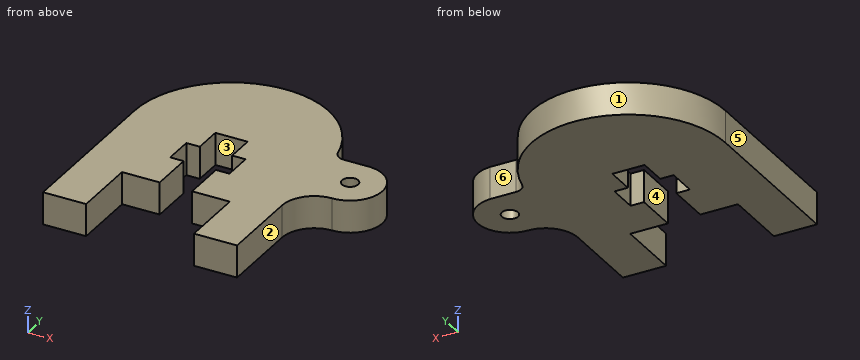
from build123d import *

# Parameters (mm, degrees)
SKETCH_1_R      = 0.75
EXTRUDE_1_DEPTH = 3


with BuildPart() as part:
    # 草图1 → 凸台-拉伸1 (new body)
    with BuildSketch(Plane.XY):
        with BuildLine():
            Line((0, 0), (4, 0))
            Line((4, 0), (4, 6))
            Line((4, 6), (7.5, 6))
            Line((7.5, 6), (7.5, 10))
            Line((7.5, 10), (6.25, 10))
            Line((6.25, 10), (6.25, 12.7))
            Line((6.25, 12.7), (7.5, 12.7))
            Line((7.5, 12.7), (7.5, 15.3))
            Line((7.5, 15.3), (10.5, 15.3))
            Line((10.5, 15.3), (10.5, 12.7))
            Line((10.5, 12.7), (11.75, 12.7))
            Line((11.75, 12.7), (11.75, 10))
            Line((11.75, 10), (10.5, 10))
            Line((10.5, 10), (10.5, 6))
            Line((10.5, 6), (14, 6))
            Line((14, 6), (14, 0))
            Line((14, 0), (18, 0))
            Line((18, 0), (18, 7.5))
            ThreePointArc((18, 7.5), (18.878679656, 9.621320344), (21, 10.5))
            ThreePointArc((21, 10.5), (23.998598833, 13.408321005), (21.183272352, 16.494396641))
            Line((21.183272352, 16.494396641), (18.756260727, 16.494396641))
            ThreePointArc((18.756260727, 16.494396641), (18.131536654, 16.713551053), (17.780634655, 17.274956977))
            ThreePointArc((17.780634655, 17.274956977), (8.006448766, 24.24499055), (0, 15.3))
            Line((0, 15.3), (0, 0))
        make_face()
        with Locations((21, 13.5)):
            Circle(SKETCH_1_R, mode=Mode.SUBTRACT)
    extrude(amount=EXTRUDE_1_DEPTH)


solid = part.part
Design review of the part built by this model. Coordinates are the model's own, in mm. Face numbers are marked on the shaded views. A direction names the side the tool comes from. Coordinates: 2 decimals unless noted, no trailing zeros. Loops run counter-clockwise (first coordinate to the right, second up) from the corner with the lowest first, then second, coordinate; pieces in that order, holes last. Notation, with made-up numbers: (2.25, 81) -> (22.25, 81) arc R29 cw to (22.25, 101) -> close; hole circle Ø1 at (1, 60.25). An arc over 180 degrees is marked (long way). Use a Markdown table: item, result. Add a question column.
Item 1: We need section C-C, the plane z = 1.9. Write out the cut boundary in (x, y).
Item 2: We need section B-B, the plane x = 6.75. Write out the cut boundary in (y, z).
Item 3: The part is to be moulded in two halves that separate along X. For the marked faces 4, 5 and 6, say which applies: +X half, -X half, draft (parallel to the pull), parting line (faces both ways), or undercut.
Item 4: We need section D-D, the plane y = 13.5. Write out the cut boundary in (x, z), and give its area (3 significant figures).
Item 5: Clearance check with flat-ended pins moving along their axes: P1, Ø0.6, axis at x = 6.5, z = 1, coming from the +Y side; P2, Ø0.6, axis at x = 7, z = 1.5, coming from the -Y side; P3, Ø1.2, axis at x = 20, z = 2, coming from the +Y side. State where each tip first meets the part, or that it passes through.
Item 6: Machinability: for the marked faces 1, 2 and 3, which of the approach directions +Z, -Z, +X, -X, +Y, -Y give a long, thin tool a straight path to every point of the face, cutting with its end or side? Answer none if there is none.
Item 7: We need section A-A, the plane y = 5. Write out the cut boundary in (x, z), and give its area (3 significant figures).
Item 8: Wall thickness on L1, parallel to Y at x = 21, z = 0.8; L2, parallel to X at y = 7.25, z = 2.3; L3, parallel to X at y = 5, z = 0.55: over which ranges is each line inside the solid? List them lowest first. Write a range as from..to.
Numbers:
| question | item | result |
|---|---|---|
| 1 | outline | (0, 0) -> (4, 0) -> (4, 6) -> (7.5, 6) -> (7.5, 10) -> (6.25, 10) -> (6.25, 12.7) -> (7.5, 12.7) -> (7.5, 15.3) -> (10.5, 15.3) -> (10.5, 12.7) -> (11.75, 12.7) -> (11.75, 10) -> (10.5, 10) -> (10.5, 6) -> (14, 6) -> (14, 0) -> (18, 0) -> (18, 7.5) arc R3 cw to (21, 10.5) arc R3 ccw to (21.18, 16.49) -> (18.76, 16.49) arc R1 cw to (17.78, 17.27) arc R9 ccw to (0, 15.3) -> close; hole circle Ø1.5 at (21, 13.5) |
| 2 | outline | (6, 0) -> (10, 0) -> (10, 3) -> (6, 3) -> close; (12.7, 0) -> (24.01, 0) -> (24.01, 3) -> (12.7, 3) -> close |
| 3 | face 4 | undercut |
| 3 | face 5 | -X half |
| 3 | face 6 | draft |
| 4 | outline | (0, 0) -> (7.5, 0) -> (7.5, 3) -> (0, 3) -> close; (10.5, 0) -> (20.25, 0) -> (20.25, 3) -> (10.5, 3) -> close; (21.75, 0) -> (24, 0) -> (24, 3) -> (21.75, 3) -> close |
| 4 | area | 58.5 mm^2 |
| 5 | P1 | stops at y = 24.03 |
| 5 | P2 | stops at y = 6 |
| 5 | P3 | stops at y = 16.49 |
| 6 | face 1 | +Z, -Z, +Y |
| 6 | face 2 | +Z, -Z, +X, -Y |
| 6 | face 3 | +Z, -Z, -Y |
| 7 | outline | (0, 0) -> (4, 0) -> (4, 3) -> (0, 3) -> close; (14, 0) -> (18, 0) -> (18, 3) -> (14, 3) -> close |
| 7 | area | 24.0 mm^2 |
| 8 | L1 | y = 10.5..12.75, 14.25..16.49 |
| 8 | L2 | x = 0..7.5, 10.5..18 |
| 8 | L3 | x = 0..4, 14..18 |
